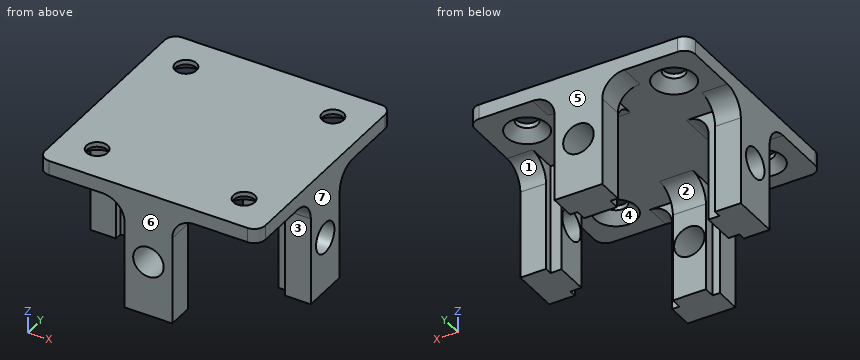
```python
from build123d import *

# Parameters (mm, degrees)
SKETCH1_W                                            = 3
SKETCH1_H                                            = 9
SKETCH1_W_2                                          = 9
SKETCH1_H_2                                          = 3
BOSS_EXTRUDE1_DEPTH                                  = 4
SKETCH1_3_W                                          = 9
SKETCH1_3_H                                          = 3
SKETCH1_3_W_2                                        = 3
SKETCH1_3_H_2                                        = 9
BOSS_EXTRUDE2_DEPTH                                  = 30
CSK_FOR_M5_HEX_SOCKET_COUNTERSUNK_CAP_SC_D           = 5.8
CSK_FOR_M5_HEX_SOCKET_COUNTERSUNK_CAP_SC_DEPTH       = 4
CSK_FOR_M5_HEX_SOCKET_COUNTERSUNK_CAP_SC_CSINK_D     = 11.2
CSK_FOR_M5_HEX_SOCKET_COUNTERSUNK_CAP_SC_CSINK_ANGLE = 90
CSK_FOR_M5_HEX_SOCKET_COUNTERSUNK_CAP_SC_TIP         = 1.742495795
FILLET1_R                                            = 3
FILLET2_R                                            = 6
CUT_EXTRUDE1_REACH                                   = 87.184
SKETCH8_R                                            = 4.15
CIRPATTERN1_COUNT                                    = 4


with BuildPart() as part:
    # Sketch1 → Boss-Extrude1 (new body)
    with BuildSketch(Plane.XY):
        Polygon((-52.5, 16), (-52.5, -7.5), (-29, -7.5), (-29, -0.5), (-27, -0.5), (-27, 2.5), (-18, 2.5), (-18, -0.5), (-16, -0.5), (-16, -7.5), (7.5, -7.5), (7.5, 16), (0.5, 16), (0.5, 18), (-2.5, 18), (-2.5, 27), (0.5, 27), (0.5, 29), (7.5, 29), (7.5, 52.5), (-16, 52.5), (-16, 45.5), (-18, 45.5), (-18, 42.5), (-27, 42.5), (-27, 45.5), (-29, 45.5), (-29, 52.5), (-52.5, 52.5), (-52.5, 29), (-45.5, 29), (-45.5, 27), (-42.5, 27), (-42.5, 18), (-45.5, 18), (-45.5, 16), align=None)
        Polygon((-52.5, 29), (-52.5, 16), (-45.5, 16), (-45.5, 18), (-45.5, 27), (-45.5, 29), align=None)
        with Locations((-44, 22.5)):
            Rectangle(SKETCH1_W, SKETCH1_H)
        Polygon((-16, 52.5), (-29, 52.5), (-29, 45.5), (-27, 45.5), (-18, 45.5), (-16, 45.5), align=None)
        with Locations((-22.5, 44)):
            Rectangle(SKETCH1_W_2, SKETCH1_H_2)
        with Locations((-1, 22.5)):
            Rectangle(SKETCH1_W, SKETCH1_H)
        Polygon((0.5, 16), (7.5, 16), (7.5, 29), (0.5, 29), (0.5, 27), (0.5, 18), align=None)
        with Locations((-22.5, 1)):
            Rectangle(SKETCH1_W_2, SKETCH1_H_2)
        Polygon((-29, -0.5), (-29, -7.5), (-16, -7.5), (-16, -0.5), (-18, -0.5), (-27, -0.5), align=None)
    extrude(amount=BOSS_EXTRUDE1_DEPTH)

    # Sketch1_3 → Boss-Extrude2 (add)
    with BuildSketch(Plane.XY):
        Polygon((-29, -0.5), (-29, -7.5), (-16, -7.5), (-16, -0.5), (-18, -0.5), (-27, -0.5), align=None)
        with Locations((-22.5, 1)):
            Rectangle(SKETCH1_3_W, SKETCH1_3_H)
        Polygon((-52.5, 29), (-52.5, 16), (-45.5, 16), (-45.5, 18), (-45.5, 27), (-45.5, 29), align=None)
        with Locations((-44, 22.5)):
            Rectangle(SKETCH1_3_W_2, SKETCH1_3_H_2)
        with Locations((-22.5, 44)):
            Rectangle(SKETCH1_3_W, SKETCH1_3_H)
        Polygon((-16, 52.5), (-29, 52.5), (-29, 45.5), (-27, 45.5), (-18, 45.5), (-16, 45.5), align=None)
        Polygon((0.5, 16), (7.5, 16), (7.5, 29), (0.5, 29), (0.5, 27), (0.5, 18), align=None)
        with Locations((-1, 22.5)):
            Rectangle(SKETCH1_3_W_2, SKETCH1_3_H_2)
    extrude(amount=-BOSS_EXTRUDE2_DEPTH)

    # CSK for M5 Hex Socket Countersunk Cap Sc
    with Locations(Plane(origin=(0, 0, 0), x_dir=(-1, 0, 0), z_dir=(0, 0, -1))):
        with Locations((2.5, 42.5), (42.5, 42.5), (42.5, 2.5), (2.5, 2.5)):
            CounterSinkHole(CSK_FOR_M5_HEX_SOCKET_COUNTERSUNK_CAP_SC_D / 2, CSK_FOR_M5_HEX_SOCKET_COUNTERSUNK_CAP_SC_CSINK_D / 2, depth=CSK_FOR_M5_HEX_SOCKET_COUNTERSUNK_CAP_SC_DEPTH, counter_sink_angle=CSK_FOR_M5_HEX_SOCKET_COUNTERSUNK_CAP_SC_CSINK_ANGLE)
            with Locations((0, 0, -(CSK_FOR_M5_HEX_SOCKET_COUNTERSUNK_CAP_SC_DEPTH + CSK_FOR_M5_HEX_SOCKET_COUNTERSUNK_CAP_SC_TIP / 2))):  # 118° drill point
                Cone(0, CSK_FOR_M5_HEX_SOCKET_COUNTERSUNK_CAP_SC_D / 2, CSK_FOR_M5_HEX_SOCKET_COUNTERSUNK_CAP_SC_TIP, mode=Mode.SUBTRACT)

    # Fillet1
    fillet1_edges = [part.edges().sort_by_distance(p)[0] for p in [
        (7.5, -7.5, 2),
        (-52.5, -7.5, 2),
        (-52.5, 52.5, 2),
        (7.5, 52.5, 2),
    ]]
    fillet(fillet1_edges, radius=FILLET1_R)

    # Fillet2
    fillet2_edges = [part.edges().sort_by_distance(p)[0] for p in [
        (-29, -4, 0),
        (-22.5, 2.5, 0),
        (-16, -4, 0),
        (-49, 29, 0),
        (-42.5, 22.5, 0),
        (-49, 16, 0),
        (-22.5, 42.5, 0),
        (-16, 49, 0),
        (-29, 49, 0),
        (4, 16, 0),
        (-2.5, 22.5, 0),
        (4, 29, 0),
    ]]
    fillet(fillet2_edges, radius=FILLET2_R)

    # Sketch8 → Cut-Extrude1 (cut, up to next)
    with BuildSketch(Plane(origin=(7.5, 0, 0), x_dir=(0, 0, -1), z_dir=(1, 0, 0)), mode=Mode.PRIVATE) as cut_extrude1_sk1:
        with Locations((15, 22.5)):
            Circle(SKETCH8_R)
    cut_extrude1_tool1 = extrude(cut_extrude1_sk1.sketch, amount=-CUT_EXTRUDE1_REACH, mode=Mode.PRIVATE) & part.part
    cut_extrude1 = cut_extrude1_tool1.solids().sort_by_distance((7.5, 22.5, -15))[0]
    add(cut_extrude1, mode=Mode.SUBTRACT)

    # CirPattern1: Cut-Extrude1 ×4 about axis
    cirpattern1_axis = Axis((-22.5, 22.5, 0), (0, 0, -1))
    for i in range(1, CIRPATTERN1_COUNT):
        add(cut_extrude1.rotate(cirpattern1_axis, i * 360 / CIRPATTERN1_COUNT), mode=Mode.SUBTRACT)


solid = part.part
```
The listing builds one solid part. Answer for the finished solid, in the listing's coordinates (mm). Face numbers are marked on the shaded views. A direction names the side the tool comes from. Give positions to 0.01 mm unless a question says otherwise; leave off trailing zeros. Order: outer loops, then holes, each group sorted by start corner. A loop starts at its lowest first (then second) coordinate and runs counter-clockwise, first axis right, second up. Notation, with made-up numbers: (42, 44.25) -> (56, 44.25) arc R26 cw to (56, 66.25) -> close; hole circle Ø10 at (68, 64). An arc over 180 degrees is marked (long way). One line per item, written item: value.
1) Flat-ended cylindrical pins translate along their axes: P1, Ø13.5, axis at x = -22.5, z = -15, coming from the -Y side; P2, Ø5, axis at y = 22.5, z = -15, coming from the +X side; P3, Ø1, axis at x = -39, y = 23.5, coming from the -Z side; P4, Ø10, axis at y = 2, z = -16.5, coming from the +X side. Find the tip coordinate at first contact, or state that the pin passes through.
Reported:
P1: stops at y = -7.5
P2: passes through
P3: stops at z = -0.8
P4: stops at x = -16
2) Find the intervals of material crossed by line 1 (X direction, y = 42.5, z = 3.1); line 2 (Y direction, x = -42.5, z = 3.1); line 3 (Y direction, x = 1, z = -15), in increasing order.
Reported:
line 1: x = -52.5 to -45.4, -39.6 to -5.4, 0.4 to 7.5
line 2: y = -7.5 to -0.4, 5.4 to 39.6, 45.4 to 52.5
line 3: y = 16 to 18.35, 26.65 to 29
3) Find section C-C, the plane x = -21.5. Determine the outline of the cut face in (y, z).
Reported:
outline: (-7.5, -30) -> (2.5, -30) -> (2.5, -19.03) -> (-7.5, -19.03) -> close; (-7.5, -10.97) -> (2.5, -10.97) -> (2.5, -6) arc R6 cw to (8.5, 0) -> (36.5, 0) arc R6 cw to (42.5, -6) -> (42.5, -10.97) -> (52.5, -10.97) -> (52.5, 4) -> (-7.5, 4) -> close; (42.5, -30) -> (52.5, -30) -> (52.5, -19.03) -> (42.5, -19.03) -> close
4) A tool of negligible diameter and unlimited length cuts with its end or side. For the marked faces 1, 2 and 3, from which of +Z, -Z, +X, -X, +Y, -Y can it reach the whole face along a straight path? Write none if from no direction.
Reported:
face 1: -Z, +X, -X, +Y
face 2: -Z, +X, -X
face 3: -Z, +X, -X, -Y
5) Find section A-A, the plane y = 22.5. Determine the outline of the cut face in (x, z).
Reported:
outline: (-52.5, -30) -> (-42.5, -30) -> (-42.5, -19.15) -> (-52.5, -19.15) -> close; (-52.5, -10.85) -> (-42.5, -10.85) -> (-42.5, -6) arc R6 cw to (-36.5, 0) -> (-8.5, 0) arc R6 cw to (-2.5, -6) -> (-2.5, -10.85) -> (7.5, -10.85) -> (7.5, 4) -> (-52.5, 4) -> close; (-2.5, -30) -> (7.5, -30) -> (7.5, -19.15) -> (-2.5, -19.15) -> close
6) Determine the mould class of the marked faces 4, 5, 6 and 7 for opening direction Y: pulls with the +Y half, pulls with the -Y half, needs draft (parallel to the pull), parting line crosses it, or undercut.
Reported:
face 4: undercut
face 5: pulls with the +Y half
face 6: pulls with the -Y half
face 7: needs draft
7) Find section D-D, the plane z = 1. Determine the outline of the cut face in (x, y).
Reported:
outline: (-52.5, -4.5) arc R3 ccw to (-49.5, -7.5) -> (4.5, -7.5) arc R3 ccw to (7.5, -4.5) -> (7.5, 49.5) arc R3 ccw to (4.5, 52.5) -> (-49.5, 52.5) arc R3 ccw to (-52.5, 49.5) -> close; hole circle Ø9.2 at (-42.5, 2.5); hole circle Ø9.2 at (-42.5, 42.5); hole circle Ø9.2 at (-2.5, 2.5); hole circle Ø9.2 at (-2.5, 42.5)
8) Find section B-B, the plane z = -24.5. Count the separate pieces of the cut face and the enclosed holes in it, plus the area to 3 significant figures.
Reported:
separate pieces: 4
enclosed holes: 0
area: 472 mm^2
